from build123d import *

# Parameters (mm, degrees)
SKETCH_1_W          = 40
SKETCH_1_H          = 40
EXTRUDE_1_DEPTH     = 3
SKETCH_2_R          = 1.5
CUT_EXTRUDE_1_DEPTH = 3
SKETCH_3_W          = 40
SKETCH_3_H          = 2
EXTRUDE_2_DEPTH     = 47


with BuildPart() as part:
    # 草图1 → 凸台-拉伸1 (new body)
    with BuildSketch(Plane.XY):
        with Locations((20, -20)):
            Rectangle(SKETCH_1_W, SKETCH_1_H)
    extrude(amount=EXTRUDE_1_DEPTH)

    # 草图2 → 切除-拉伸1 (cut)
    with BuildSketch(Plane.XY.offset(3)):
        with Locations((35, -8)):
            Circle(SKETCH_2_R)
        with Locations(Location((5, -8, 0), (0, 0, 180))):
            Circle(SKETCH_2_R)
        with Locations((35, -32)):
            Circle(SKETCH_2_R)
        with Locations(Location((5, -32, 0), (0, 0, 180))):
            Circle(SKETCH_2_R)
    extrude(amount=-CUT_EXTRUDE_1_DEPTH, mode=Mode.SUBTRACT)

    # 草图3 → 凸台-拉伸2 (add)
    with BuildSketch(Plane.XY.offset(3)):
        with Locations((20, -39)):
            Rectangle(SKETCH_3_W, SKETCH_3_H)
    extrude(amount=EXTRUDE_2_DEPTH)


solid = part.part
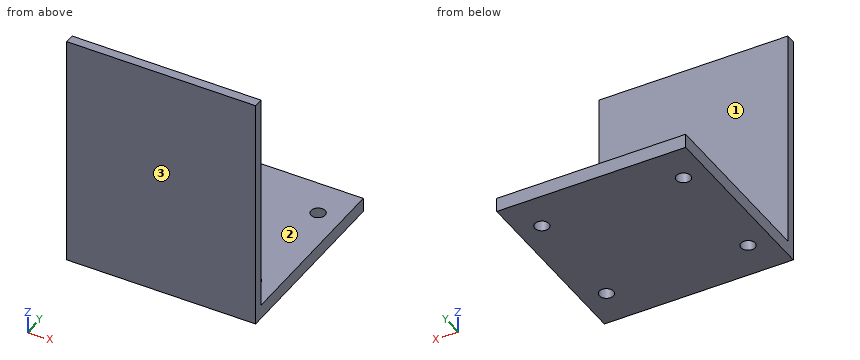
The model under review builds one solid part; all positions refer to its coordinate system, in mm. Face numbers are marked on the shaded views. Round coordinates to 2 decimals unless told otherwise and drop trailing zeros. Loops run counter-clockwise (first coordinate to the right, second up) from the corner with the lowest first, then second, coordinate; pieces in that order, holes last. Notation, with made-up numbers: M 52.5,32 L 95.5,32 A33 ccw 95.5,64 Z; hole C 12.25,70 d1. An arc over 180 degrees is marked long. Answer as CSV lines item,"result". Start each with the question number.
Item 1: Consider section A-A (x = 35). Write out the cut boundary in (y, z), then the cut area to 3 significant figures.
Item 2: Mouldability with a two-part tool opening along Y and no side actions: class the marked faces 1, 2 and 3 as released by +Y, released by -Y, zero draft, split by the parting line, or undercut.
Item 3: Insertion check: P1, Ø3, axis at x = 23, z = 16.5, coming from the +Y side; P2, Ø11.5, axis at x = 23.5, y = -24.5, coming from the +Z side. Each pin has a flat end and moves straight along its axis. Give the tip position at first contact, or say it passes through.
Item 4: Consider section B-B (y = -8). Write out the cut boundary in (x, z), then the cut area to 3 significant figures.
Item 5: Wall thickness on line 1 (Y direction, x = 5, z = 1.45); line 2 (Z direction, x = 2.5, y = -6); line 3 (Y direction, x = 25, z = 48.5): over which ranges is each line inside the solid? List them lowest first. Write a range as [from, to].
Item 6: Consider section D-D (y = -14). Write out the cut boundary in (x, z), then the cut area to 3 significant figures.
Item 7: Consider section C-C (x = 24). Write out the cut boundary in (y, z), then the cut area to 3 significant figures.
Answer:
1,outline,"M -40,0 L -33.5,0 L -33.5,3 L -38,3 L -38,50 L -40,50 Z; M -30.5,0 L -9.5,0 L -9.5,3 L -30.5,3 Z; M -6.5,0 L 0,0 L 0,3 L -6.5,3 Z"
1,area,"196 mm^2"
2,face 1,"released by +Y"
2,face 2,"zero draft"
2,face 3,"released by -Y"
3,P1,"stops at y = -38"
3,P2,"stops at z = 3"
4,outline,"M 0,0 L 3.5,0 L 3.5,3 L 0,3 Z; M 6.5,0 L 33.5,0 L 33.5,3 L 6.5,3 Z; M 36.5,0 L 40,0 L 40,3 L 36.5,3 Z"
4,area,"102 mm^2"
5,line 1,"y = [-40, -33.5], [-30.5, -9.5], [-6.5, 0]"
5,line 2,"z = [0, 3]"
5,line 3,"y = [-40, -38]"
6,outline,"M 0,0 L 40,0 L 40,3 L 0,3 Z"
6,area,"120 mm^2"
7,outline,"M -40,0 L 0,0 L 0,3 L -38,3 L -38,50 L -40,50 Z"
7,area,"214 mm^2"
